Model file for the job. Use its own axes, mm. A direction names the side the tool comes from. Give positions to 0.01 mm unless a question says otherwise; leave off trailing zeros. Loops run counter-clockwise (first coordinate to the right, second up) from the corner with the lowest first, then second, coordinate; pieces in that order, holes last. Notation, with made-up numbers: M -1,23 L 8,23 A25 ccw 8,45 Z; hole C -18,-2.5 d11. An arc over 180 degrees is marked long. Answer in a Markdown table with one row per item.
```python
from build123d import *

# Parameters (mm, degrees)
PAD_DEPTH    = 2
PAD001_DEPTH = 51
PAD002_DEPTH = 5
PAD003_DEPTH = 5


with BuildPart() as part:
    # Sketch → Pad (new body)
    with BuildSketch(Plane.XY):
        with BuildLine():
            Line((-15, 13), (-15, -13))
            ThreePointArc((-15, -13), (-14.414214, -14.414214), (-13, -15))
            Line((-13, -15), (13, -15))
            ThreePointArc((13, -15), (14.414214, -14.414214), (15, -13))
            Line((15, -13), (15, 13))
            ThreePointArc((15, 13), (14.414214, 14.414214), (13, 15))
            Line((13, 15), (-13, 15))
            ThreePointArc((-13, 15), (-14.414214, 14.414214), (-15, 13))
        make_face()
    extrude(amount=PAD_DEPTH)

    # Sketch001 (on Face10 of Pad) → Pad001 (join)
    with BuildSketch(Plane.XY.offset(2)):
        with BuildLine():
            Line((-15, 13), (-15, -13))
            ThreePointArc((-15, -13), (-14.414214, -14.414214), (-13, -15))
            Line((-13, -15), (13, -15))
            ThreePointArc((13, -15), (14.414214, -14.414214), (15, -13))
            Line((15, -13), (15, 13))
            ThreePointArc((15, 13), (14.414214, 14.414214), (13, 15))
            Line((13, 15), (-13, 15))
            ThreePointArc((-13, 15), (-14.414214, 14.414214), (-15, 13))
        make_face()
        with BuildLine():
            Line((-14, 12), (-14, -12))
            ThreePointArc((-14, -12), (-13.414214, -13.414214), (-12, -14))
            Line((-12, -14), (12, -14))
            ThreePointArc((12, -14), (13.414214, -13.414214), (14, -12))
            Line((14, -12), (14, 12))
            ThreePointArc((14, 12), (13.414214, 13.414214), (12, 14))
            Line((12, 14), (-12, 14))
            ThreePointArc((-12, 14), (-13.414214, 13.414214), (-14, 12))
        make_face(mode=Mode.SUBTRACT)
    extrude(amount=PAD001_DEPTH)

    # Sketch002 (on Face13 of Pad001) → Pad002 (join)
    with BuildSketch(Plane(origin=(0, 15, 0), x_dir=(-1, 0, 0), z_dir=(0, 1, 0))):
        with BuildLine():
            ThreePointArc((2.2, 50.8), (0, 53), (-2.2, 50.8))
            Line((-2.2, 50.8), (-2.2, 48.7))
            ThreePointArc((-2.2, 48.7), (0, 46.5), (2.2, 48.7))
            Line((2.2, 50.8), (2.2, 48.7))
        make_face()
        with BuildLine():
            ThreePointArc((-2.2, 8.7), (0, 6.5), (2.2, 8.7))
            Line((2.2, 8.7), (2.2, 10.8))
            ThreePointArc((2.2, 10.8), (0, 13), (-2.2, 10.8))
            Line((-2.2, 8.7), (-2.2, 10.8))
        make_face()
    extrude(amount=PAD002_DEPTH)

    # Sketch003 (on Face28 of Pad002) → Pad003 (join)
    with BuildSketch(Plane(origin=(0, 20, 0), x_dir=(-1, 0, 0), z_dir=(0, 1, 0))):
        with BuildLine():
            ThreePointArc((2.2, 50.8), (0, 53), (-2.2, 50.8))
            Line((-2.2, 50.8), (-2.2, 42.2))
            ThreePointArc((-2.2, 42.2), (0, 40), (2.2, 42.2))
            Line((2.2, 50.8), (2.2, 42.2))
        make_face()
        with BuildLine():
            ThreePointArc((2.2, 10.8), (0, 13), (-2.2, 10.8))
            Line((-2.2, 10.8), (-2.2, 2.2))
            ThreePointArc((-2.2, 2.2), (0, 0), (2.2, 2.2))
            Line((2.2, 10.8), (2.2, 2.2))
        make_face()
    extrude(amount=PAD003_DEPTH)


solid = part.part
```
(1) Mould opens along X. For faces 1 (the cylindrical face through (0, 20, 53)), 2 (the flat face through (-14, 0, 27)), 3 (the flat face through (0, 20, 3)), 4 (the flat face through (0, -14, 27)) say: pulls with the +X half, pulls with the -X half, needs draft (parallel to the pull), parting line crosses it, or undercut.
Established:
| item | result |
|---|---|
| face 1 | parting line crosses it |
| face 2 | undercut |
| face 3 | needs draft |
| face 4 | undercut |
(2) Saw through at A-A, the plane z = 45.5. Give the cut face in (x, y).
Established:
| item | result |
|---|---|
| outline | M -15,-13 A2 ccw -13,-15 L 13,-15 A2 ccw 15,-13 L 15,13 A2 ccw 13,15 L -13,15 A2 ccw -15,13 Z; M -2.2,20 L 2.2,20 L 2.2,25 L -2.2,25 Z; hole M -14,-12 A2 ccw -12,-14 L 12,-14 A2 ccw 14,-12 L 14,12 A2 ccw 12,14 L -12,14 A2 ccw -14,12 Z |
(3) Saw through at C-C, the plane z = 32. Give the cut face in (x, y), and give its area (3 significant figures).
Established:
| item | result |
|---|---|
| outline | M -15,-13 A2 ccw -13,-15 L 13,-15 A2 ccw 15,-13 L 15,13 A2 ccw 13,15 L -13,15 A2 ccw -15,13 Z; hole M -14,-12 A2 ccw -12,-14 L 12,-14 A2 ccw 14,-12 L 14,12 A2 ccw 12,14 L -12,14 A2 ccw -14,12 Z |
| area | 116 mm2 |
(4) Wall check: L1, parallel to Y at x = 1.5, z = 46; L2, parallel to Y at x = 5, z = 13. Give the ranges that are in metal, low to high.
Established:
| item | result |
|---|---|
| L1 | y = -15 to -14, 14 to 15, 20 to 25 |
| L2 | y = -15 to -14, 14 to 15 |
(5) Flat gauge pins, fed straight in: P1, Ø9.5, axis at y = 21, z = 47, coming from the +X side; P2, Ø9.5, axis at y = 19.5, z = 45.5, coming from the -X side; P3, Ø7, axis at y = 18, z = 7, coming from the -X side; P4, Ø10, axis at y = 15, z = 31, coming from the -X side. Where does each tip first touch, or does it go through?
Established:
| item | result |
|---|---|
| P1 | stops at x = 2.2 |
| P2 | stops at x = -13.97 |
| P3 | stops at x = -14.32 |
| P4 | stops at x = -15 |
(6) Saw through at B-B, the plane y = -3. Give the cut face in (x, z).
Established:
| item | result |
|---|---|
| outline | M -15,0 L 15,0 L 15,53 L 14,53 L 14,2 L -14,2 L -14,53 L -15,53 Z |
(7) Which spindle directions (+Z, -Z, +X, -X, +Y, -Y) get a long thin tool onto all of the face, cutting with end or side? Do faces 5 (the flat face through (2.2, 22, 7)), 6 (the cylindrical face through (13.43, 13.4, 27.14)), 7 (the flat face through (-2.2, 22, 7)). Say none if no direction does.
Established:
| item | result |
|---|---|
| face 5 | +Z, -Z, +X, +Y |
| face 6 | +Z |
| face 7 | +Z, -Z, -X, +Y |
